```python
from build123d import *

# Parameters (mm, degrees)
BOX016_W                  = 16
BOX016_H                  = 34
BOX016_DEPTH              = 90
BOX016_PLACEMENT_ANGLE    = 45
FILLET_R                  = 7
FILLET001_R               = 2
FILLET001_PLACEMENT_ANGLE = 90


with BuildPart() as part:
    # Box016 → Box016 (new body)
    with BuildSketch(Plane.XY):
        with Locations((8, 17)):
            Rectangle(BOX016_W, BOX016_H)
    extrude(amount=BOX016_DEPTH)


with BuildPart() as part_1:
    # Box016 placement: moved
    add(part.part.moved(Location((0, 0, 180))).rotate(Axis((0, 0, 180), (0, 0, 1)), BOX016_PLACEMENT_ANGLE))

    # Fillet
    fillet_edges = [part_1.edges().sort_by_distance(p)[0] for p in [
        (-12.020815, 12.020815, 270),
        (-12.020815, 12.020815, 180),
        (-0.707107, 23.334524, 270),
        (-0.707107, 23.334524, 180),
    ]]
    fillet(fillet_edges, radius=FILLET_R)


with BuildPart() as part_2:
    # Fillet placement: moved
    add(part_1.part.moved(Location((-2, -26, -162))))

    # Fillet001
    fillet001_edges = [part_2.edges().sort_by_distance(p)[0] for p in [
        (-2, -26, 63),
        (-26.041631, -1.958369, 63),
    ]]
    fillet(fillet001_edges, radius=FILLET001_R)


with BuildPart() as part_3:
    # Fillet001 placement: moved
    add(part_2.part.rotate(Axis((0, 0, 0), (0, 0, 1)), FILLET001_PLACEMENT_ANGLE))


solid = part_3.part
```
Source: CAD feature listing. Evaluate the final solid. Frame: model axes, mm. Coordinates: 2 decimals unless noted, no trailing zeros. Write each loop counter-clockwise with the first axis right and the second up, starting at its lowest first coordinate (ties: lowest second). Pieces come first, ordered by that corner, then holes. Notation, with made-up numbers: M 43.25,78 L 71.25,78 A6 ccw 71.25,86 Z; hole C -6.5,52.25 d6. An arc over 180 degrees is marked long. Answer as a JSON object with one key per item and string values.
1. Cut plane A-A on z = 48. Output: boundary loops of the cut face in (x, y).
Evaluation:
{"outline": "M -7.94,-16.14 L 0.54,-24.63 A2 ccw 3.37,-24.63 L 24.59,-3.41 A2 ccw 24.59,-0.59 L 16.1,7.9 A2 ccw 13.27,7.9 L -7.94,-13.31 A2 ccw Z"}
2. Ray query, L1, parallel to Y at x = 15.5, z = 74; L2, parallel to Z at x = 12, y = -3; L3, parallel to Y at x = -1, z = 47. Return the intervals inside material, ascending.
Evaluation:
{"L1": "-12.5 to 8.31", "L2": "18 to 108", "L3": "-23.08 to -6.37"}
3. Contact query for flat-ended pins moving along their axis: P1, Ø5, axis at y = -20, z = 58.5, coming from the +X side; P2, Ø5, axis at x = -4, z = 41, coming from the -Y side; P3, Ø5, axis at x = 7, z = 42.5, coming from the -Y side. Output: stop coordinate, or through.
Evaluation:
{"P1": "x = 10.5", "P2": "y = -22.58", "P3": "y = -23.5"}
